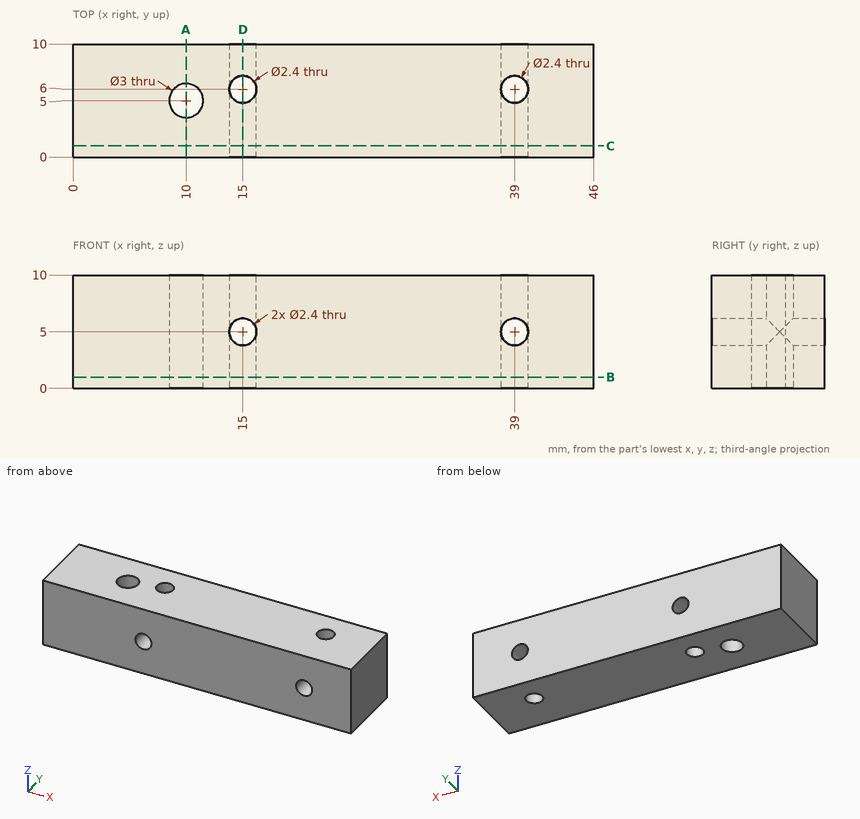
Could you check a few things on this drawing? It's one solid part, dimensions in mm from its lowest x, y, z. Give positions to 0.01 mm unless a question says otherwise; leave off trailing zeros. Write each loop counter-clockwise with the first axis right and the second up, starting at its lowest first coordinate (ties: lowest second). Pieces come first, ordered by that corner, then holes. Notation, with made-up numbers: (48.5, 71) -> (68.5, 71) arc R12 cw to (68.5, 91) -> close; hole circle Ø4 at (22, 57.5). An arc over 180 degrees is marked (long way). Write item = value, one per line.
(1) Suppose I cut it at C-C on y = 1. Write out the boundary of the cut face in (x, z).
Worked out:
outline = (0, 0) -> (46, 0) -> (46, 10) -> (0, 10) -> close; hole circle Ø2.4 at (15, 5); hole circle Ø2.4 at (39, 5)
(2) Suppose I cut it at D-D on x = 15. Write out the boundary of the cut face in (y, z).
Worked out:
outline = (0, 0) -> (4.8, 0) -> (4.8, 3.8) -> (0, 3.8) -> close; (0, 6.2) -> (4.8, 6.2) -> (4.8, 10) -> (0, 10) -> close; (7.2, 0) -> (10, 0) -> (10, 3.8) -> (7.2, 3.8) -> close; (7.2, 6.2) -> (10, 6.2) -> (10, 10) -> (7.2, 10) -> close
(3) Suppose I cut it at A-A on x = 10. Write out the boundary of the cut face in (y, z).
Worked out:
outline = (0, 0) -> (3.5, 0) -> (3.5, 10) -> (0, 10) -> close; (6.5, 0) -> (10, 0) -> (10, 10) -> (6.5, 10) -> close
(4) Suppose I cut it at B-B on z = 1. Write out the boundary of the cut face in (x, y).
Worked out:
outline = (0, 0) -> (46, 0) -> (46, 10) -> (0, 10) -> close; hole circle Ø3 at (10, 5); hole circle Ø2.4 at (15, 6); hole circle Ø2.4 at (39, 6)
(5) I need wall thicknesses on probe 1 along X at (y, z) = (9.1, 5); probe 2 along X at (y, z) = (5.5, 7); probe 3 along Y at (x, z) = (15, 8.9). Which ranges of each line are inside material? Lowest first, please. Write a range as from..to.
Worked out:
probe_1 = 0..13.8, 16.2..37.8, 40.2..46
probe_2 = 0..8.59, 11.41..13.91, 16.09..37.91, 40.09..46
probe_3 = 0..4.8, 7.2..10
